```python
from build123d import *

# Parameters (mm, degrees)
SKETCH1_R           = 4
BOSS_EXTRUDE1_DEPTH = 10
SKETCH2_R           = 7.5
BOSS_EXTRUDE2_DEPTH = 10
SKETCH3_W           = 2.232233047
SKETCH3_H           = 0.5
CUT_EXTRUDE1_DEPTH  = 0.1
SKETCH6_R           = 7.5
BOSS_EXTRUDE5_DEPTH = 10
SKETCH7_W           = 50
SKETCH7_H           = 6
BOSS_EXTRUDE6_DEPTH = 3


with BuildPart() as part:
    # Sketch1 → Boss-Extrude1 (new body)
    with BuildSketch(Plane.XY):
        Circle(SKETCH1_R)
    extrude(amount=BOSS_EXTRUDE1_DEPTH)

    # Sketch2 → Boss-Extrude2 (add)
    with BuildSketch(Plane.XY.offset(10)):
        with Locations((2, 0)):
            Circle(SKETCH2_R)
    extrude(amount=BOSS_EXTRUDE2_DEPTH)

    # Sketch3 → Cut-Extrude1 (cut)
    with BuildSketch(Plane.XY.offset(20)):
        Polygon((-1.5, 0.5), (-0.232233047, 0.5), (-0.232233047, 1.767766953), align=None)
        Polygon((-2, 0), (-0.232233047, 0), (-0.232233047, 0.5), (-1.5, 0.5), align=None)
        Polygon((-0.232233047, -0.5), (-0.232233047, 0), (-2, 0), (-1.5, -0.5), align=None)
        Polygon((-0.232233047, -1.767766953), (-0.232233047, -0.5), (-1.5, -0.5), align=None)
        with Locations((0.883883476, 0.25)):
            Rectangle(SKETCH3_W, SKETCH3_H)
        with Locations((0.883883476, -0.25)):
            Rectangle(SKETCH3_W, SKETCH3_H)
    extrude(amount=-CUT_EXTRUDE1_DEPTH, mode=Mode.SUBTRACT)

    # Sketch6 → Boss-Extrude5 (add)
    with BuildSketch(Plane.XY.offset(20)):
        with Locations(Location((-0.034904813, 1.99969539, 0), (0, 0, 236.464463187))):
            Circle(SKETCH6_R)
    extrude(amount=BOSS_EXTRUDE5_DEPTH)

    # Sketch7 → Boss-Extrude6 (add)
    with BuildSketch(Plane(origin=(0, 0, 0), x_dir=(-1, 0, 0), z_dir=(0, 0, -1))):
        with Locations((25, 0)):
            Rectangle(SKETCH7_W, SKETCH7_H)
    extrude(amount=-BOSS_EXTRUDE6_DEPTH)


solid = part.part
```
For this review, take the finished solid that the model builds, in its own axes (mm). A direction names the side the tool comes from. Give positions to 0.01 mm unless a question says otherwise; leave off trailing zeros. Write each loop counter-clockwise with the first axis right and the second up, starting at its lowest first coordinate (ties: lowest second). Pieces come first, ordered by that corner, then holes. Notation, with made-up numbers: M -12,-28.75 L 25,-28.75 A31 cw 25,6.25 Z; hole C 60,23.5 d5. An arc over 180 degrees is marked long. Answer as a JSON object with one key per item and string values. Group by question number.
Item 1: For probe 1 along Z at (x, y) = (-24.5, 0); probe 2 along Z at (x, y) = (-4, -1.25); probe 3 along Y at (x, z) = (0, 6.75), list the stretches that pass through material, from the lowest coordinate up. Write a range as [from, to].
Item 2: Consider section C-C on y = 5.25. Write out the cut boundary in (x, z), plus the area to 3 significant figures.
Item 3: For pin 1 Ø5 at (y, z) = (1, 10) entering from +X; pin 2 Ø5 at (x, y) = (-17, 1) entering from +Z; pin 3 Ø1.5 at (x, z) = (-15, 2) entering from -Y; pin 4 Ø3.5 at (x, z) = (-18.5, 1) entering from +Y, all flat-tipped, find the tip position at first contact; note any pin that passes through.
Item 4: Consider section B-B on z = 7.5. Write out the cut boundary in (x, y), plus the area to 3 significant figures.
Item 5: Consider section A-A on x = -14. Write out the cut boundary in (y, z).
Item 6: Draft analysis for pull direction Z (two halves, no side actions). For faces 1 (the flat face through (-23, 0, 0)), 2 (the flat face through (-26, -3, 1)), 3 (the cylindrical face through (3.695, -1.532, 4.93)), state which applies: +Z half, -Z half, draft (parallel to the pull), parting line (faces both ways), or undercut.
Item 7: Tool access review of faces 4 (the cylindrical face through (3.009, -4.855, 24.93)), 5 (the flat face through (-50, 0, 1)): name each direction out of +Z, -Z, +X, -X, +Y, -Y from which nothing blocks a thin tool from reaching the whole face with its end or side.
Check result:
{
 "1": {"probe 1": "z = [0, 3]", "probe 2": "z = [0, 3], [10, 30]", "probe 3": "y = [-4, 4]"},
 "2": {"outline": "M -6.79,20 L -3.36,20 L -3.36,10 L 7.36,10 L 7.36,20 L 6.72,20 L 6.72,30 L -6.79,30 Z", "area": "242 mm^2"},
 "3": {"pin 1": "stops at x = 9.5", "pin 2": "stops at z = 3", "pin 3": "stops at y = -3", "pin 4": "stops at y = 3"},
 "4": {"outline": "C 0,0 d8", "area": "50.3 mm^2"},
 "5": {"outline": "M -3,0 L 3,0 L 3,3 L -3,3 Z"},
 "6": {"face 1": "-Z half", "face 2": "draft", "face 3": "undercut"},
 "7": {"face 4": "+Z", "face 5": "+Z, -Z, -X, +Y, -Y"}
}
